Model file for the job. Use its own axes, mm. A direction names the side the tool comes from. Round coordinates to 2 decimals unless told otherwise and drop trailing zeros. Loops run counter-clockwise (first coordinate to the right, second up) from the corner with the lowest first, then second, coordinate; pieces in that order, holes last. Notation, with made-up numbers: M -0.75,-0.5 L 11.25,-0.5 A35 ccw 11.25,36.5 Z; hole C 25,-34.5 d11. An arc over 180 degrees is marked long. Use a Markdown table: item, result. Add a question column.
Q1. Pin check, flat tips, straight feed: pin 1 (10 mm diameter, centred on x = -11, z = 12, fed in from +Y); pin 2 (6.5 mm diameter, centred on x = -1.5, y = 27, fed in from +Z); pin 3 (0.9 mm diameter, centred on x = -1, z = 4, fed in from +Y). Stop position of each tip, or through.
Q2. Cut at B-B (x = 0). Give the cut face in (y, z), plus the area to 3 significant figures.
Q3. Cut at A-A (z = -6.5). Give the cut face in (x, y), plus the area to 3 significant figures.
Q4. Tool access for faces 4 (the face through (-7, 0, 4)), 5 (the face through (-3, 21.5, 6.4)), 6 (the face through (0, 23, 9)), 7 (the face through (0, 10, 5)), 8 (the face through (0, 23, 0)): list every direction of +Z, -Z, +X, -X, +Y, -Y with a clear straight run to the whole face (end or side of a thin tool).
Q5. Probe line 1 (Y direction, x = 0, z = 7.5); line 2 (Y direction, x = -4.5, z = 13.5); line 3 (X direction, y = 38.75, z = 6.6). List the from-to ranges inside material, lowest first. Write a range as from..to.
Q6. Cut at C-C (z = 8). Give the cut face in (x, y).
Q7. Mould opens along Y. For faces 1 (the face through (0.231, 38.306, 7.521)), 2 (the face through (-0.1, 41.5, 7.5)), 3 (the face through (0, 26, 6)) say: +Y half, -Y half, draft (parallel to the pull), parting line (faces both ways), or undercut.
Q8. Cut at D-D (y = 3). Give the cut face in (x, z), plus the area to 3 significant figures.
Autodesk Inventor part; units mm, degrees
ref_plane "YZ Plane" through (0, 0, 0) normal (1, 0, 0) x (0, 1, 0)
ref_plane "XZ Plane" through (0, 0, 0) normal (0, 1, 0) x (-1, 0, 0)
ref_plane "XY Plane" through (0, 0, 0) normal (0, 0, 1) x (1, 0, 0)
sketch "Sketch1" plane through (0, 0, 0) normal (0, 0, 1) x (1, 0, 0)
  line L0 (-3, 38.5) -> (-3, 0)
  line L1 (-3, 0) -> (3, 0)
  line L2 (3, 0) -> (3, 38.5)
  line L3 (-3, 38.5) -> (-3, 36)
  arc A0 (3, 38.5) -> (-3, 38.5) centre (0, 38.5) ccw
  point P0 (0, 0)
extrude "Extrusion1" add sketch "Sketch1" along normal blind 9
sketch "Sketch2" plane through (3, 0, 0) normal (1, 0, 0) x (0, 0, -1)
  line L0 (-3, 41.5) -> (-6, 41.5)
  line L1 (-6, 41.5) -> (-6, 10)
  line L2 (-6, 10) -> (-3, 10)
  line L3 (-3, 10) -> (-3, 41.5)
  point P0 (0, 0)
  point P1 (-9, 41.5)
extrude "Extrusion2" cut sketch "Sketch2" against normal through all
sketch "Sketch3" plane through (0, 0, 9) normal (0, 0, 1) x (1, 0, 0)
  line L0 (-3, 38.5) -> (-3, 0)
  line L1 (-3, 4) -> (3, 4)
  line L2 (3, 0) -> (-17, 0)
  line L3 (-17, 0) -> (-17, 4)
  line L4 (-17, 4) -> (3, 4)
  line L5 (3, 0) -> (3, 4)
  line L6 (3, 0) -> (3, 38.5)
  point P0 (0, 0)
  dimension "d77" = 20
sketch "Sketch8" plane through (0, 0, 9) normal (0, 0, 1) x (1, 0, 0)
  arc A0 (3, 38.5) -> (-3, 38.5) centre (0, 38.5) ccw construction
  line L0 (0, 41.5) -> (0, 38.75) construction
  circle A1 centre (0, 38.75) radius 0.5
  point P0 (0, 0)
  dimension "d68" = 2.75
  dimension "d69" = 1
extrude "Extrusion6" cut sketch "Sketch8" against normal through all
extrude "Extrusion7" add sketch "Sketch3" along normal blind 13.5 and the other way blind 22.5
sketch "Sketch10" plane through (-3, 4, 9) normal (0, 1, 0) x (1, 0, 0)
  point P0 (3, 9)
  point P1 (6, 22.5)
  point P2 (6, -13.5)
  point P3 (-4.142, -6.5)
  point P4 (-4.142, 15.5)
hole "Hole4" at (-7.142, 4, 15.5) at (-7.142, 4, -6.5) direction (0, -1, 0) diameter 3.4 end through all
properties part number "Podstawka" material "Stainless Steel, Austenitic"
Checked values:
| question | item | result |
|---|---|---|
| 1 | pin 1 | stops at y = 4 |
| 1 | pin 2 | stops at z = 9 |
| 1 | pin 3 | stops at y = 10 |
| 2 | outline | M 0,-13.5 L 4,-13.5 L 4,0 L 38.25,0 L 38.25,3 L 10,3 L 10,6 L 38.25,6 L 38.25,9 L 4,9 L 4,22.5 L 0,22.5 Z; M 39.25,0 L 41.5,0 L 41.5,3 L 39.25,3 Z; M 39.25,6 L 41.5,6 L 41.5,9 L 39.25,9 Z |
| 2 | area | 381 mm^2 |
| 3 | outline | M -17,0 L -8.84,0 L -8.84,4 L -17,4 Z; M -5.44,0 L 3,0 L 3,4 L -5.44,4 Z |
| 3 | area | 66.4 mm^2 |
| 4 | face 4 | +Z, -Z, +X, -X, -Y |
| 4 | face 5 | +Z, -Z, -X, +Y |
| 4 | face 6 | +Z, +X, -X, +Y |
| 4 | face 7 | +X, -X, +Y |
| 4 | face 8 | -Z, +X, -X, +Y |
| 5 | line 1 | y = 0..38.25, 39.25..41.5 |
| 5 | line 2 | y = 0..4 |
| 5 | line 3 | x = -2.99..-0.5, 0.5..2.99 |
| 6 | outline | M -17,0 L 3,0 L 3,38.5 A3 ccw -3,38.5 L -3,4 L -17,4 Z; hole C 0,38.75 d1 |
| 7 | face 1 | undercut |
| 7 | face 2 | +Y half |
| 7 | face 3 | draft |
| 8 | outline | M -17,-13.5 L 3,-13.5 L 3,22.5 L -17,22.5 Z; hole C -7.14,-6.5 d3.4; hole C -7.14,15.5 d3.4 |
| 8 | area | 702 mm^2 |
